from build123d import *

# Parameters (mm, degrees)
F1_DEPTH = 533.4
F3_DEPTH = 30.48
F5_DEPTH = 25.4


with BuildPart() as f1:
    # F0 (on Front) → F1 (new body)
    with BuildSketch(Plane.XZ):
        Polygon((-20.0246775488, 194.6782106813), (-248.6246775488, 194.6782106813), (-248.6246775488, 100.6982106813), (-223.2246775488, 100.6982106813), (-224.7843856167, -140.0887378329), (-223.2246775488, -155.8417893187), (-45.4246775488, -155.8417893187), (-43.8649694809, -140.0887378329), (-45.4246775488, 100.6982106813), (-20.0246775488, 100.6982106813), align=None)
        Polygon((-223.2246775488, 100.6982106813), (-248.6246775488, 100.6982106813), (-224.7843856167, -140.0887378329), align=None)
        Polygon((-43.8649694809, -140.0887378329), (-20.0246775488, 100.6982106813), (-45.4246775488, 100.6982106813), align=None)
    extrude(amount=F1_DEPTH)

    # F2 (on face) → F3 (cut)
    with BuildSketch(Plane.XZ.offset(533.4)):
        Polygon((-223.0825424194, 100.6982106813), (-248.6246775488, 100.6982106813), (-223.2246775488, -155.8417893187), align=None)
        Polygon((-45.4246775488, 100.6982106813), (-45.4246775488, -155.8417893187), (-20.0246775488, 100.6982106813), align=None)
    extrude(amount=-F3_DEPTH, mode=Mode.SUBTRACT)

    # F4 (on face) → F5 (cut)
    with BuildSketch(Plane.XZ):
        Polygon((-43.5820221101, -153.1578327248), (-18.1820221101, 100.8364513063), (-20.0246775488, 100.8364513063), (-20.0246775488, 100.6982106813), (-45.2851133126, 100.6982106813), align=None)
        Polygon((-223.2246775488, 100.6982106813), (-246.6658660559, 100.6982106813), (-224.6561073752, -120.2852073061), align=None)
        Polygon((-222.1963950907, 100.6689677848), (-246.7820221101, 101.8644461788), (-246.6658660559, 100.6982106813), (-223.2246775488, 100.6982106813), (-224.6561073752, -120.2852073061), (-221.3820221101, -153.1578327248), align=None)
    extrude(amount=-F5_DEPTH, mode=Mode.SUBTRACT)


solid = f1.part
The model under review builds one solid part; all positions refer to its coordinate system, in mm. A direction names the side the tool comes from. Coordinates: 2 decimals unless noted, no trailing zeros. Write each loop counter-clockwise with the first axis right and the second up, starting at its lowest first coordinate (ties: lowest second). Pieces come first, ordered by that corner, then holes. Notation, with made-up numbers: M 65.25,-38.5 L 107.25,-38.5 A25 ccw 107.25,-3.5 Z; hole C -19.75,-13.5 d1. An arc over 180 degrees is marked long. Put each result on its own line as item: value.
1) Add section C-C on z = 34. Give the boundary of the cut face in (x, y).
Computed:
outline: M -242.02,-502.92 L -223.12,-502.92 L -223.12,-533.4 L -45.42,-533.4 L -45.42,-502.92 L -26.63,-502.92 L -26.63,0 L -242.02,0 Z
2) Draft analysis for pull direction Z (two halves, no side actions). For faces 4 (the flat face through (-36, -502.92, 3)), 5 (the flat face through (-133, -263, 194.678)), 6 (the flat face through (-32.902, -247.94, -29.368)), state which applies: released by +Z, released by -Z, zero draft, split by the parting line, or undercut.
Computed:
face 4: zero draft
face 5: released by +Z
face 6: released by -Z
3) Add section A-A on z = -106. Give the boundary of the cut face in (x, y).
Computed:
outline: M -228.16,-502.92 L -223.2,-502.92 L -223.2,-533.4 L -45.42,-533.4 L -45.42,-502.92 L -40.49,-502.92 L -40.49,0 L -228.16,0 Z
4) Add section B-B on y = -381. Give the boundary of the cut face in (x, z), then the cut area to 3 significant figures.
Computed:
outline: M -248.62,100.7 L -223.22,-155.84 L -45.42,-155.84 L -20.02,100.7 L -20.02,194.68 L -248.62,194.68 Z
area: 73,600 mm2
5) Wall thickness on probe 1 along X at (y, z) = (-284, 46); probe 2 along X at (y, z) = (-58, -12.5): over which ranges is each line inside the solid? List them lowest first. Write a range as [from, to].
Computed:
probe 1: x = [-243.21, -25.44]
probe 2: x = [-237.42, -31.23]
6) Clearance check with flat-ended pins moving along their axes: pin 1 Ø12 at (y, z) = (-391, 78) entering from +X; pin 2 Ø3 at (y, z) = (-247, 16) entering from +X; pin 3 Ø7.5 at (x, y) = (-27.5, -519.5) entering from -Z; pin 4 Ø12 at (x, z) = (-49, -59.5) entering from +Y. State where each tip first meets the part, or that it passes through.
Computed:
pin 1: stops at x = -21.68
pin 2: stops at x = -28.26
pin 3: stops at z = 100.7
pin 4: stops at y = 0
7) For faces 1 (the flat face through (-136, 0, 22)), 2 (the flat face through (-236, -518, 100.698)), 3 (the flat face through (-33, -518, 100.698)), list the 3-axis set-ups (+Z, -Z, +X, -X, +Y, -Y) from which the entire face can be reached by the end or side of a thin tool; tool diameter is ignored.
Computed:
face 1: +Z, -Z, +X, -X, +Y
face 2: -Z, -X, -Y
face 3: -Z, +X, -Y
